```python
from build123d import *

# Parameters (mm, degrees)
F0_W      = 1200
F0_H      = 570
F1_DEPTH  = 18
F3_DEPTH  = 300
F4_W      = 1200
F4_H      = 570
F5_DEPTH  = 18
F6_W      = 700
F6_H      = 570
F7_DEPTH  = 18
F8_W      = 18
F8_H      = 570
F9_DEPTH  = 764
F10_W     = 682
F10_H     = 570
F10_W_2   = 18
F11_DEPTH = 18
F12_W     = 18
F12_H     = 570
F13_DEPTH = 764
F14_W     = 270
F14_H     = 18
F14_W_2   = 376
F15_DEPTH = 570


with BuildPart() as f1:
    # F0 (on Top) → F1 (new body)
    with BuildSketch(Plane.XY):
        Rectangle(F0_W, F0_H)
    extrude(amount=F1_DEPTH)

    # F2 (on face) → F3 (join)
    with BuildSketch(Plane.XY.offset(18)):
        Polygon((-582, 285), (-600, 285), (-600, -285), (-582, -285), (-582, 92.4397557974), align=None)
        Polygon((-188, 285), (-206, 285), (-206, 92.4397557974), (-206, -285), (-188, -285), (-188, 93.6823561788), align=None)
        Polygon((206, 285), (188, 285), (188, 93.6823561788), (188, -285), (206, -285), (206, 93.6823785305), align=None)
        Polygon((600, 285), (582, 285), (582, 93.6823785305), (582, -285), (600, -285), align=None)
    extrude(amount=F3_DEPTH)

    # F4 (on face) → F5 (join)
    with BuildSketch(Plane.XY.offset(318)):
        Rectangle(F4_W, F4_H)
    extrude(amount=F5_DEPTH)

    # F6 (on face) → F7 (join)
    with BuildSketch(Plane.XY.offset(336)):
        with Locations((-250, 0)):
            Rectangle(F6_W, F6_H)
    extrude(amount=F7_DEPTH)

    # F8 (on face) → F9 (join)
    with BuildSketch(Plane.XY.offset(354)):
        with Locations((-591, 0)):
            Rectangle(F8_W, F8_H)
        with Locations((91, 0)):
            Rectangle(F8_W, F8_H)
    extrude(amount=F9_DEPTH)

    # F10 (on face) → F11 (join)
    with BuildSketch(Plane.XY.offset(1118)):
        with Locations((-259, 0)):
            Rectangle(F10_W, F10_H)
        with Locations((91, 0)):
            Rectangle(F10_W_2, F10_H)
    extrude(amount=F11_DEPTH)

    # F12 (on face) → F13 (join)
    with BuildSketch(Plane.XY.offset(354)):
        with Locations((-197, 0)):
            Rectangle(F12_W, F12_H)
    extrude(amount=F13_DEPTH)

    # F14 (on face) → F15 (join)
    with BuildSketch(Plane.XZ.offset(285)):
        with Locations((-53, 736)):
            Rectangle(F14_W, F14_H)
        with Locations((-394, 867)):
            Rectangle(F14_W_2, F14_H)
        with Locations((-394, 607)):
            Rectangle(F14_W_2, F14_H)
    extrude(amount=-F15_DEPTH)


solid = f1.part
```
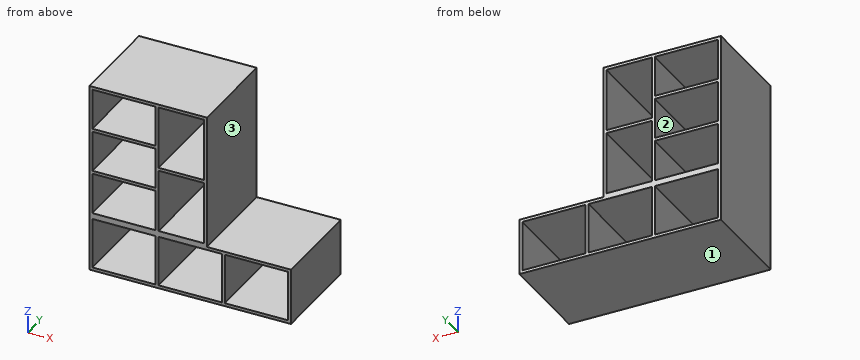
Geometry check sheet. Reference: the model listing, model coordinates, mm. Face numbers are marked on the shaded views. Coordinates: 2 decimals unless noted, no trailing zeros. Write each loop counter-clockwise with the first axis right and the second up, starting at its lowest first coordinate (ties: lowest second). Pieces come first, ordered by that corner, then holes. Notation, with made-up numbers: M -37.5,29 L -24.5,29 A18 ccw -24.5,42 Z; hole C 88,0.25 d1. An arc over 180 degrees is marked long. Use one line per item in the form item = value. Start each with the question number.
1) Go/stop test with flat-tipped pins: pin 1 Ø8 at (x, y) = (423, 150) entering from +Z; pin 2 Ø5 at (y, z) = (21.5, 852) entering from +X. Record where each tip stops, or that it passes through.
2) Section check B-B on z = 381.5. Enter the section's corners in (x, y), and give its area (3 significant figures).
3) Section check C-C on x = 424. Enter the section's corners in (y, z), and give its area (3 significant figures).
4) Section check D-D on x = -50. Enter the section's corners in (y, z), and give its area (3 significant figures).
5) Thickness scan on probe 1 along X at (y, z) = (218, 258); probe 2 along X at (y, z) = (249, 816); probe 3 along Z at (x, y) = (-446, 94.5). Record the ranges inside material, lowest first. Write a range as from..to.
6) Section check A-A on x = -387. Enter the section's corners in (y, z), and give its area (3 significant figures).
7) Release check for a two-part mould opening along X. For the marked faces 1, 2 and 3 record: pulls with the +X half, pulls with the -X half, needs draft (parallel to the pull), parting line crosses it, or undercut.
Responses:
q1.pin_1 = 336
q1.pin_2 = 100
q2.outline = M -600,-285 L -582,-285 L -582,285 L -600,285 Z; M -206,-285 L -188,-285 L -188,285 L -206,285 Z; M 82,-285 L 100,-285 L 100,285 L 82,285 Z
q2.area = 30,800 mm2
q3.outline = M -285,0 L 285,0 L 285,18 L -285,18 Z; M -285,318 L 285,318 L 285,336 L -285,336 Z
q3.area = 20,500 mm2
q4.outline = M -285,0 L 285,0 L 285,18 L -285,18 Z; M -285,318 L 285,318 L 285,354 L -285,354 Z; M -285,727 L 285,727 L 285,745 L -285,745 Z; M -285,1118 L 285,1118 L 285,1136 L -285,1136 Z
q4.area = 51,300 mm2
q5.probe_1 = -600..-582, -206..-188, 188..206, 582..600
q5.probe_2 = -600..-582, -206..-188, 82..100
q5.probe_3 = 0..18, 318..354, 598..616, 858..876, 1118..1136
q6.outline = M -285,0 L 285,0 L 285,18 L -285,18 Z; M -285,318 L 285,318 L 285,354 L -285,354 Z; M -285,598 L 285,598 L 285,616 L -285,616 Z; M -285,858 L 285,858 L 285,876 L -285,876 Z; M -285,1118 L 285,1118 L 285,1136 L -285,1136 Z
q6.area = 61,600 mm2
q7.face_1 = needs draft
q7.face_2 = undercut
q7.face_3 = pulls with the +X half
